Part model, mm, in its own coordinate system. A direction names the side the tool comes from. Give positions to 0.01 mm unless a question says otherwise; leave off trailing zeros. Order: outer loops, then holes, each group sorted by start corner. A loop starts at its lowest first (then second) coordinate and runs counter-clockwise, first axis right, second up.
from build123d import *

# Parameters (mm, degrees)
SKETCH1_R           = 7
BOSS_EXTRUDE1_DEPTH = 30
SKETCH2_R           = 12.5
SKETCH2_R_2         = 1.5
BOSS_EXTRUDE2_DEPTH = 3


with BuildPart() as part:
    # Sketch1 → Boss-Extrude1 (new body)
    with BuildSketch(Plane(origin=(0, 0, 0), x_dir=(0, 0, -1), z_dir=(1, 0, 0))):
        Circle(SKETCH1_R)
    extrude(amount=-BOSS_EXTRUDE1_DEPTH)

    # Sketch2 → Boss-Extrude2 (add)
    with BuildSketch(Plane(origin=(0, 0, 0), x_dir=(0, 0, -1), z_dir=(1, 0, 0))):
        Circle(SKETCH2_R)
        with Locations((0, 9.94711279)):
            Circle(SKETCH2_R_2, mode=Mode.SUBTRACT)
        with Locations((9.94711279, 0)):
            Circle(SKETCH2_R_2, mode=Mode.SUBTRACT)
        with Locations((0, -9.94711279)):
            Circle(SKETCH2_R_2, mode=Mode.SUBTRACT)
        with Locations((-9.94711279, 0)):
            Circle(SKETCH2_R_2, mode=Mode.SUBTRACT)
    extrude(amount=BOSS_EXTRUDE2_DEPTH)


solid = part.part
Item 1: Band-saw the part on C-C on z = 7.5. List the corners of the cut face in (x, y).
Item 2: Which spindle directions (+Z, -Z, +X, -X, +Y, -Y) get a long thin tool onto all of the face, cutting with end or side? Do faces 1 (the face through (0, -5.4, -5.4)), 2 (the face through (1.48, -11.41, 0.33)). Say none if no direction does.
Item 3: Band-saw the part on D-D on y = -5.75. List the corners of the cut face in (x, z).
Item 4: Drill centre lines: probe 1 along Y at (x, z) = (1.45, 0); probe 2 along Z at (x, y) = (-9.5, 0.25); probe 3 along X at (y, z) = (6.75, 2.25). Where is each one in solid material? Low to high.
Item 5: Drop flat-ended pins along their axis: P1, Ø2.5, axis at y = 9.95, z = 0, coming from the +X side; P2, Ø10, axis at x = -15.5, y = 4.5, coming from the -Z side; P3, Ø1, axis at x = -20, y = 5.5, coming from the -Z side; P4, Ø12, axis at x = -1, y = -3, coming from the -Z side. Give the stop position or say it passes through.
Item 6: Band-saw the part on A-A on z = 0. List the corners of the cut face in (x, y).
Item 7: Pull direction Z, two halves, no side cores. Call faces 3 (the face through (1.479, 0.066, 11.446)), 4 (the face through (1.48, 11.21, -0.81)), 5 (the face through (-14.79, -2.681, -6.466)), 6 (the face through (3, 0, 0)): released by +Z, released by -Z, zero draft, split by the parting line, or undercut.
Working result:
1. outline: (0, -10) - (3, -10) - (3, 10) - (0, 10) - close
2. face 1: -X
2. face 2: +X, -X
3. outline: (-30, -3.99) - (0, -3.99) - (0, -11.1) - (3, -11.1) - (3, 11.1) - (0, 11.1) - (0, 3.99) - (-30, 3.99) - close
4. probe 1: y = -12.5 to -11.45, -8.45 to 8.45, 11.45 to 12.5
4. probe 2: z = -7 to 7
4. probe 3: x = 0 to 3
5. P1: passes through
5. P2: stops at z = -7
5. P3: stops at z = -4.9
5. P4: stops at z = -12.5
6. outline: (-30, -7) - (0, -7) - (0, -8.45) - (3, -8.45) - (3, 8.45) - (0, 8.45) - (0, 7) - (-30, 7) - close; (0, -12.5) - (3, -12.5) - (3, -11.45) - (0, -11.45) - close; (0, 11.45) - (3, 11.45) - (3, 12.5) - (0, 12.5) - close
7. face 3: undercut
7. face 4: undercut
7. face 5: split by the parting line
7. face 6: zero draft
